Design review of the part built by this model. Coordinates are the model's own, in mm. Round coordinates to 2 decimals unless told otherwise and drop trailing zeros. Write each loop counter-clockwise with the first axis right and the second up, starting at its lowest first coordinate (ties: lowest second). Pieces come first, ordered by that corner, then holes. Notation, with made-up numbers: (37.5, 65.5) -> (73.5, 65.5) arc R26 ccw to (73.5, 98.5) -> close; hole circle Ø5 at (22, -13). An arc over 180 degrees is marked (long way). Write item = value, one per line. Start each with the question number.
Item 1: To check wall thickness, follow L1, parallel to X at y = 2.45, z = 30; L2, parallel to X at y = 2.7, z = -25; L3, parallel to Z at x = 12.5, y = 1.15. State the ranges of each line that lie inside material, in increasing order.
Item 2: Add section A-A, the plane y = 0.65. State how many separate pieces and enclosed holes the cut face has, then the cut area to 3 significant figures.
Item 3: For pin 1 Ø1.2 at (x, y) = (13.5, 1.5) entering from -Z; pin 2 Ø1.5 at (x, y) = (-8, 2) entering from -Z, all flat-tipped, find the tip position at first contact; note any pin that passes through.
Item 4: Mouldability with a two-part tool opening along Z and no side actions: class faces 1 (the cylindrical face through (-16.15, 1.97, -24.97)), 2 (the flat face through (0, 4, 1)) as released by +Z, released by -Z, zero draft, split by the parting line, or undercut.
Item 5: Add section B-B, the plane z = -29.5. State the section outline as (x, y) points.
Autodesk Fusion 360 part; units mm, degrees
sketch "Sketch1" plane through (0, 0, 0) normal (0, 1, 0) x (1, 0, 0)
  line L0 (-17.5, 25) -> (-17.5, -25)
  line L1 (17.5, -25) -> (17.5, 25)
  circle A0 centre (0, 25) radius 0.5
  arc A1 (17.5, 25) -> (-17.5, 25) centre (0, 25) ccw
  line L2 (-15, 23.85) -> (-9, 23.85)
  arc A2 (-9, 23.85) -> (-9, 26.15) centre (-9, 25) ccw
  line L3 (-9, 26.15) -> (-15, 26.15)
  arc A3 (-15, 26.15) -> (-15, 23.85) centre (-15, 25) ccw
  line L4 (-15, 25) -> (-9, 25) construction
  circle A4 centre (-12.5, -30) radius 0.5
  circle A5 centre (12.5, -30) radius 0.5
  line L5 (-17.5, -25) -> (-17.5, -45)
  line L6 (-17.5, -45) -> (17.5, -45)
  line L7 (17.5, -25) -> (17.5, -45)
  arc A6 (-14.7164, 21.8774) -> (-14.0684, 19.6706) centre (-14.3924, 20.774) ccw
  arc A7 (-8.3114, 21.361) -> (-8.9594, 23.5678) centre (-8.6354, 22.4644) ccw
  line L8 (-14.0684, 19.6706) -> (-8.3114, 21.361)
  line L9 (-8.9594, 23.5678) -> (-14.7164, 21.8774)
  line L10 (-14.3924, 20.774) -> (-8.6354, 22.4644) construction
  arc A8 (-13.2405, 17.8578) -> (-11.9971, 15.9229) centre (-12.6188, 16.8904) ccw
  arc A9 (-6.9495, 19.1668) -> (-8.193, 21.1017) centre (-7.5713, 20.1342) ccw
  line L11 (-11.9971, 15.9229) -> (-6.9495, 19.1668)
  line L12 (-8.193, 21.1017) -> (-13.2405, 17.8578)
  line L13 (-12.6188, 16.8904) -> (-7.5713, 20.1342) construction
  arc A10 (-10.692, 14.4168) -> (-8.9538, 12.9107) centre (-9.8229, 13.6638) ccw
  arc A11 (-5.0246, 17.4452) -> (-6.7629, 18.9513) centre (-5.8937, 18.1983) ccw
  line L14 (-8.9538, 12.9107) -> (-5.0246, 17.4452)
  line L15 (-6.7629, 18.9513) -> (-10.692, 14.4168)
  line L16 (-9.8229, 13.6638) -> (-5.8937, 18.1983) construction
  arc A12 (-7.2773, 11.8332) -> (-5.1851, 10.8778) centre (-6.2312, 11.3555) ccw
  arc A13 (-2.6927, 16.3356) -> (-4.7848, 17.291) centre (-3.7387, 16.8133) ccw
  line L17 (-5.1851, 10.8778) -> (-2.6927, 16.3356)
  line L18 (-4.7848, 17.291) -> (-7.2773, 11.8332)
  line L19 (-6.2312, 11.3555) -> (-3.7387, 16.8133) construction
  arc A14 (-3.273, 10.3163) -> (-0.9964, 9.989) centre (-2.1347, 10.1527) ccw
  arc A15 (-0.1425, 15.9279) -> (-2.4191, 16.2553) centre (-1.2808, 16.0916) ccw
  line L20 (-0.9964, 9.989) -> (-0.1425, 15.9279)
  line L21 (-2.4191, 16.2553) -> (-3.273, 10.3163)
  line L22 (-2.1347, 10.1527) -> (-1.2808, 16.0916) construction
  arc A16 (0.9964, 9.989) -> (3.273, 10.3163) centre (2.1347, 10.1527) ccw
  arc A17 (2.4191, 16.2553) -> (0.1425, 15.9279) centre (1.2808, 16.0916) ccw
  line L23 (3.273, 10.3163) -> (2.4191, 16.2553)
  line L24 (0.1425, 15.9279) -> (0.9964, 9.989)
  line L25 (2.1347, 10.1527) -> (1.2808, 16.0916) construction
  arc A18 (5.1851, 10.8778) -> (7.2773, 11.8332) centre (6.2312, 11.3555) ccw
  arc A19 (4.7848, 17.291) -> (2.6927, 16.3356) centre (3.7387, 16.8133) ccw
  line L26 (7.2773, 11.8332) -> (4.7848, 17.291)
  line L27 (2.6927, 16.3356) -> (5.1851, 10.8778)
  line L28 (6.2312, 11.3555) -> (3.7387, 16.8133) construction
  arc A20 (8.9538, 12.9107) -> (10.692, 14.4168) centre (9.8229, 13.6638) ccw
  arc A21 (6.7629, 18.9513) -> (5.0246, 17.4452) centre (5.8937, 18.1983) ccw
  line L29 (10.692, 14.4168) -> (6.7629, 18.9513)
  line L30 (5.0246, 17.4452) -> (8.9538, 12.9107)
  line L31 (9.8229, 13.6638) -> (5.8937, 18.1983) construction
  arc A22 (11.9971, 15.9229) -> (13.2405, 17.8578) centre (12.6188, 16.8904) ccw
  arc A23 (8.193, 21.1017) -> (6.9495, 19.1668) centre (7.5713, 20.1342) ccw
  line L32 (13.2405, 17.8578) -> (8.193, 21.1017)
  line L33 (6.9495, 19.1668) -> (11.9971, 15.9229)
  line L34 (12.6188, 16.8904) -> (7.5713, 20.1342) construction
  arc A24 (14.0684, 19.6706) -> (14.7164, 21.8774) centre (14.3924, 20.774) ccw
  arc A25 (8.9594, 23.5678) -> (8.3114, 21.361) centre (8.6354, 22.4644) ccw
  line L35 (14.7164, 21.8774) -> (8.9594, 23.5678)
  line L36 (8.3114, 21.361) -> (14.0684, 19.6706)
  line L37 (14.3924, 20.774) -> (8.6354, 22.4644) construction
  arc A26 (15, 23.85) -> (15, 26.15) centre (15, 25) ccw
  arc A27 (9, 26.15) -> (9, 23.85) centre (9, 25) ccw
  line L38 (15, 26.15) -> (9, 26.15)
  line L39 (9, 23.85) -> (15, 23.85)
  line L40 (15, 25) -> (9, 25) construction
  dimension "d1" = 50
  dimension "d2" = 35
  dimension "d4" = 1
  dimension "d7" = 15
  dimension "d31" = 2.3
  dimension "d45" = 1
  dimension "d46" = 1
  dimension "d49" = 5
  dimension "d50" = 5
  dimension "d52" = 20
  dimension "d54" = 15
  dimension "d55" = 15
  dimension "d58" = 6
  dimension "d62" = 180
extrude "Extrude4" add sketch "Sketch1" along normal blind 4
Result set:
q1.L1 = -17.5 to -13, -12 to 12, 13 to 17.5
q1.L2 = -17.5 to -16.15, -7.85 to -0.5, 0.5 to 7.85, 16.15 to 17.5
q1.L3 = -37.25 to -26.15, -23.85 to -22.53, -20.13 to -18.33, -15.75 to 29.5, 30.5 to 45
q2.separate_pieces = 1
q2.enclosed_holes = 15
q2.area = 2,710 mm²
q3.pin_1 = -36.83
q3.pin_2 = -40.93
q4.face_1 = undercut
q4.face_2 = zero draft
q5.outline = (-16.91, 0) -> (16.91, 0) -> (16.91, 4) -> (-16.91, 4) -> close
